Geometry: final body of the model. Coordinates: model frame, mm. A direction names the side the tool comes from. Round coordinates to 2 decimals unless told otherwise and drop trailing zeros. Order: outer loops, then holes, each group sorted by start corner. A loop starts at its lowest first (then second) coordinate and runs counter-clockwise, first axis right, second up. Notation, with made-up numbers: M 59.25,0.5 L 95.25,0.5 A25 ccw 95.25,24.5 Z; hole C -32,51 d10. An arc over 180 degrees is marked long. Put each result on its own line as item: value. Start each with the question number.
1) First-contact query: P1, Ø1.5, axis at x = 18, z = 21, coming from the +Y side; P2, Ø2, axis at x = 8, y = 12, coming from the +Z side; P3, Ø6, axis at x = 6, z = 10.5, coming from the -Y side; P4, Ø2.5, axis at x = 13.5, y = 21, coming from the +Z side. Flat tips, straight axial feed; report the tip coordinate or a pass-through.
2) Access query for faces 3 (the flat face through (12, 19.05, 9)), 4 (the flat face through (10, 15.875, 3)), 5 (the flat face through (13, 22, 19.05)), 6 (the flat face through (3, 19.05, 16)). Directions: +Z, -Z, +X, -X, +Y, -Y. A direction counts if a zero-diameter tool reaches every point of the face in a straight line with its end or side. Return the directions, or none.
3) Section A-A, the plane x = 12. Return loops of the section in (y, z) (3 decimals).
4) Draft query along X for faces 1 (the cylindrical face through (14.3, 17.5, 3.1)), 2 (the flat face through (22, 19.05, 23)). Return one class per face: pulls with the +X half, pulls with the -X half, needs draft (parallel to the pull), parting line crosses it, or undercut.
5) Material intervals for probe 1 along X at (y, z) = (23, 16.25); probe 2 along X at (y, z) = (7.75, 23.75), sorted ascending. Write a range as [from, to].
6) Section C-C, the plane z = 20. Return loops of the section in (x, y), then the cut area to 3 significant figures.
7) Section B-B, the plane y = 14.75. Return loops of the section in (x, z).
from build123d import *

# Parameters (mm, degrees)
F5_DEPTH = 6.35
F6_DEPTH = 6.35
F7_DEPTH = 6.35
F8_R     = 5.08


with BuildPart() as f5:
    # F2 (on Top) → F5 (new body)
    with BuildSketch(Plane.XY):
        with BuildLine():
            Line((0, 25.4), (0, 0))
            Line((0, 0), (19.05, 0))
            Line((19.05, 0), (19.05, 6.35))
            ThreePointArc((19.05, 6.35), (17.190128, 10.840128), (12.7, 12.7))
            ThreePointArc((12.7, 12.7), (17.190128, 14.559872), (19.05, 19.05))
            Line((19.05, 19.05), (19.05, 25.4))
            Line((19.05, 25.4), (0, 25.4))
        make_face()
        with BuildLine():
            Line((6.35, 6.35), (6.35, 9.525))
            Line((6.35, 9.525), (12.714883, 9.525))
            ThreePointArc((12.714883, 9.525), (14.3024, 7.930024), (12.7, 6.35))
            Line((12.7, 6.35), (6.35, 6.35))
        make_face(mode=Mode.SUBTRACT)
        with BuildLine():
            Line((6.35, 15.875), (6.35, 19.05))
            Line((6.35, 19.05), (12.7, 19.05))
            ThreePointArc((12.7, 19.05), (14.3024, 17.469976), (12.714883, 15.875))
            Line((12.714883, 15.875), (6.35, 15.875))
        make_face(mode=Mode.SUBTRACT)
    extrude(amount=F5_DEPTH)

    # F4 (on offset) → F6 (join)
    with BuildSketch(Plane.YZ.offset(25.4)):
        with BuildLine():
            Line((19.050006, -0.00045), (25.400006, -0.00045))
            Line((25.400006, -0.00045), (25.400006, 25.39955))
            Line((25.400006, 25.39955), (19.050006, 25.39955))
            Line((19.050006, 25.39955), (19.050006, 20.614292))
            ThreePointArc((19.050006, 20.614292), (17.11549, 17.691652), (13.669329, 18.330519))
            Line((13.669329, 18.330519), (6.350006, 25.39955))
            Line((6.350006, 25.39955), (6e-06, 25.39955))
            Line((6e-06, 25.39955), (6e-06, 19.04955))
            Line((6e-06, 19.04955), (6.57484, 12.69955))
            Line((6.57484, 12.69955), (6e-06, 6.34955))
            Line((6e-06, 6.34955), (6e-06, -0.00045))
            Line((6e-06, -0.00045), (6.350006, -0.00045))
            Line((6.350006, -0.00045), (13.669329, 7.068581))
            ThreePointArc((13.669329, 7.068581), (17.11549, 7.707448), (19.050006, 4.784809))
            Line((19.050006, 4.784809), (19.050006, -0.00045))
        make_face()
    extrude(amount=-F6_DEPTH)

    # F3 (on offset) → F7 (join)
    with BuildSketch(Plane.XZ.offset(-25.4)):
        Polygon((6.35, 25.4), (0, 25.4), (0, 0), (25.4, 0), (25.4, 25.4), (19.05, 25.4), (19.05, 6.35), (15.24, 6.35), (15.24, 19.05), (10.16, 19.05), (10.16, 6.35), (6.35, 6.35), align=None)
    extrude(amount=F7_DEPTH)

    # F8
    f8_edges = [f5.edges().sort_by_distance(p)[0] for p in [
        (22.225, 6.57484, 12.69955),
    ]]
    fillet(f8_edges, radius=F8_R)


solid = f5.part
Result sheet:
1. P1: passes through
1. P2: stops at z = 6.35
1. P3: stops at y = 19.05
1. P4: stops at z = 19.05
2. face 3: +Z
2. face 4: +Z, -Z
2. face 5: +Z, +Y, -Y
2. face 6: +Z, -X, -Y
3. outline: M 0,0 L 6.35,0 L 6.35,6.35 L 0,6.35 Z; M 9.525,0 L 15.875,0 L 15.875,6.35 L 9.525,6.35 Z; M 19.05,0 L 25.4,0 L 25.4,19.05 L 19.05,19.05 Z
4. face 1: undercut
4. face 2: needs draft
5. probe 1: x = [0, 6.35], [10.16, 15.24], [19.05, 25.4]
5. probe 2: x = [19.05, 25.4]
6. outline: M 0,19.05 L 6.35,19.05 L 6.35,25.4 L 0,25.4 Z; M 19.05,0 L 25.4,0 L 25.4,11.94 L 19.05,11.94 Z; M 19.05,18.99 L 25.4,18.99 L 25.4,25.4 L 19.05,25.4 Z
6. area: 157 mm2
7. outline: M 0,0 L 17.37,0 L 17.37,6.35 L 0,6.35 Z; M 19.05,7.75 L 25.4,7.75 L 25.4,17.65 L 19.05,17.65 Z
